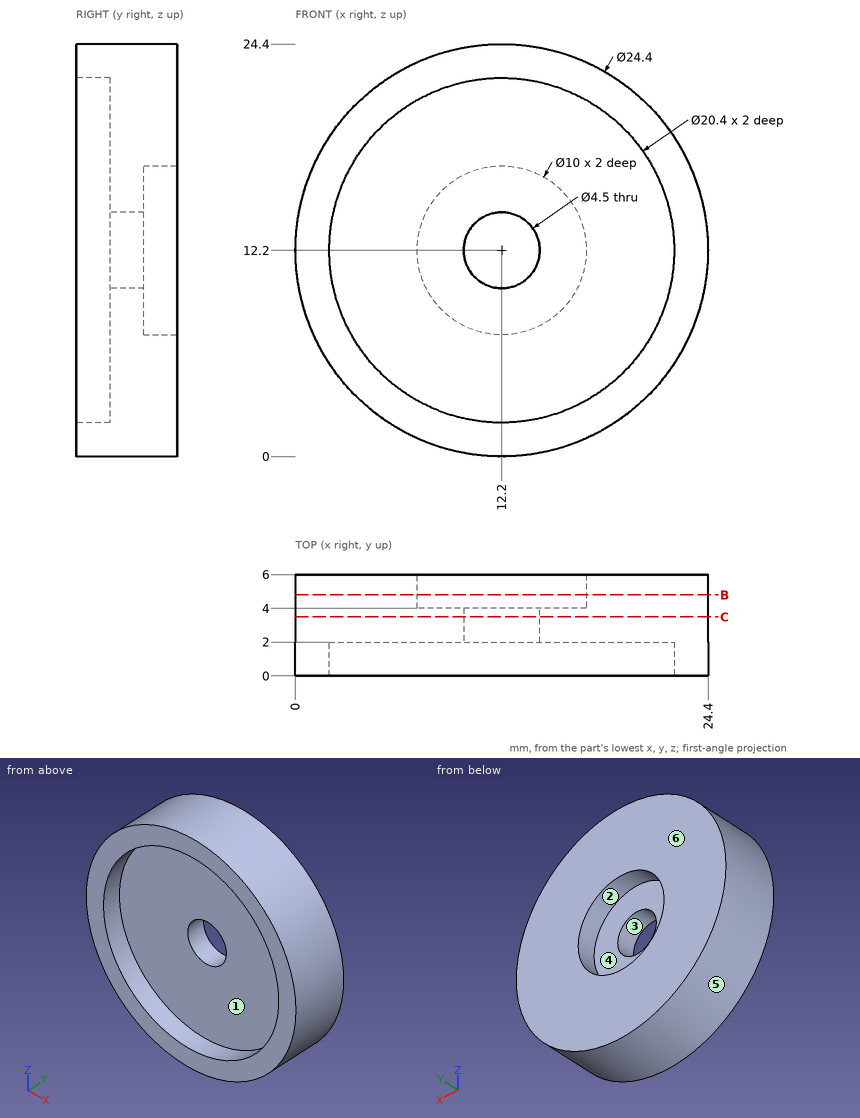
Design review of the part shown in the three views and the two pictorial views. Dimensions are in mm from the part's minimum x, y and z. A direction names the side the tool comes from. Round coordinates to 2 decimals unless told otherwise and drop trailing zeros. Order: outer loops, then holes, each group sorted by start corner. A loop starts at its lowest first (then second) coordinate and runs counter-clockwise, first axis right, second up. Notation, with made-up numbers: (-6, -29.75) - (27, -29.75) arc R10 cw to (27, -20.75) - close; hole circle Ø9 at (-25, 20). An arc over 180 degrees is marked (long way). One line per question, with ' | ' between items.
Item 1: Machinability: for the marked faces 1, 2 and 3, which of the approach directions +Z, -Z, +X, -X, +Y, -Y give a long, thin tool a straight path to every point of the face, cutting with its end or side? Answer none if there is none.
Checks:
face 1: -Y | face 2: +Y | face 3: +Y, -Y
Item 2: Draft analysis for pull direction X (two halves, no side actions). For the marked faces 4, 5 and 6, state which applies: +X half, -X half, draft (parallel to the pull), parting line (faces both ways), or undercut.
Checks:
face 4: undercut | face 5: parting line | face 6: draft
Item 3: Take a section at B-B, the plane y = 4.8. Write out the cut boundary in (x, z), then the cut area to 3 significant figures.
Checks:
outline: circle Ø24.4 at (12.2, 12.2); hole circle Ø10 at (12.2, 12.2) | area: 389 mm²
Item 4: Wall thickness on line 1 (X direction, y = 2.45, z = 12.2); line 2 (Y direction, x = 16.5, z = 5.5): over which ranges is each line inside the solid? List them lowest first. Write a range as [from, to].
Checks:
line 1: [0, 9.95], [14.45, 24.4] | line 2: [2, 6]
Item 5: For P1, Ø3, axis at x = 9, y = 4.5, coming from the -Z side; P2, Ø1.5, axis at y = 3, z = 17, coming from the -X side; P3, Ø11.5, axis at x = 12.2, z = 12.2, coming from the +Y side; P4, Ø5, axis at x = 11.5, z = 11.5, coming from the +Y side, all flat-tipped, find the tip position at first contact; note any pin that passes through.
Checks:
P1: z = 0.12 | P2: x = 0.69 | P3: y = 6 | P4: y = 4
Item 6: Take a section at C-C, the plane y = 3.5. Write out the cut boundary in (x, z).
Checks:
outline: circle Ø24.4 at (12.2, 12.2); hole circle Ø4.5 at (12.2, 12.2)
